from build123d import *

# Parameters (mm, degrees)
F0_R        = 50.8
F1_DEPTH    = 63.5
F2_T1_DEPTH = 128.3697077416
F2_T3_DEPTH = 128.3697077416
F2_T5_DEPTH = 78.8079500043


# Not quite as in the source:
# - a fillet or chamfer that OpenCascade refuses, or shapes differently, is made with other operations: its cross-section is extruded or revolved along the edge and cut away or added


with BuildPart() as f1:
    # F0 (on Top) → F1 (new body)
    with BuildSketch(Plane.XY):
        Polygon((-88.9, -51.326438931), (0, -102.6528778619), (88.9, -51.326438931), (88.9, 51.326438931), (0, 102.6528778619), (-88.9, 51.326438931), align=None)
        Circle(F0_R, mode=Mode.SUBTRACT)
    extrude(amount=F1_DEPTH)

    # F2: chamfer of 5 on 6 edges, made by hand

    # F2_s2 → F2_t1 (cut)
    with BuildSketch(Plane(origin=(55.5857139903, -32.0924269354, 0), x_dir=(0, 0, 1), z_dir=(-0.8660254038, 0.5, 0))):
        Polygon((58.5, 88.9), (63.5, 83.9), (63.5, 88.9), align=None)
        Polygon((5, 88.9), (0, 83.9), (0, 88.9), align=None)
    extrude(amount=F2_T1_DEPTH, mode=Mode.SUBTRACT)

    # F2_s4 → F2_t3 (cut)
    with BuildSketch(Plane(origin=(55.5857139903, 32.0924269354, 0), x_dir=(0, 0, 1), z_dir=(-0.8660254038, -0.5, 0))):
        Polygon((58.5, 88.9), (63.5, 83.9), (63.5, 88.9), align=None)
        Polygon((5, 88.9), (0, 83.9), (0, 88.9), align=None)
    extrude(amount=F2_T3_DEPTH, mode=Mode.SUBTRACT)

    # F2_s6 → F2_t5 (cut)
    with BuildSketch(Plane.XY.offset(-7.6539750021)):
        Polygon((-88.9, 48.439687585), (-86.4, 52.7698146039), (-88.9, 51.326438931), align=None)
        Polygon((88.9, 48.439687585), (86.4, 52.7698146039), (88.9, 51.326438931), align=None)
    extrude(amount=F2_T5_DEPTH, mode=Mode.SUBTRACT)


solid = f1.part
Work out the finished part from the listing and answer in its coordinate system (mm). Give positions to 0.01 mm unless a question says otherwise; leave off trailing zeros. Write each loop counter-clockwise with the first axis right and the second up, starting at its lowest first coordinate (ties: lowest second). Pieces come first, ordered by that corner, then holes.
Q1. The part is cut by section A-A on z = 48. Give the vertices of the cut face in (x, y).
Answer:
outline: (-88.9, -51.33) - (0, -102.65) - (88.9, -51.33) - (88.9, 48.44) - (86.4, 52.77) - (0, 102.65) - (-86.4, 52.77) - (-88.9, 48.44) - close; hole circle Ø101.6 at (0, 0)
Q2. Straight lines are drawn through the part: L1, parallel to Y at x = 0, z = 26; L2, parallel to Y at x = 39, z = 59; L3, parallel to X at y = 31, z = 54.5. For each, find the intervals that lie inside material, in ascending order.
Answer:
L1: y = -102.65 to -50.8, 50.8 to 102.65
L2: y = -80.14 to -32.55, 32.55 to 79.56
L3: x = -88.9 to -40.24, 40.24 to 88.9
Q3. The part is cut by section C-C on x = -12.5. Give the vertices of the cut face in (y, z).
Answer:
outline: (-95.44, 0) - (-49.24, 0) - (-49.24, 63.5) - (-95.44, 63.5) - close; (49.24, 0) - (89.66, 0) - (95.44, 5) - (95.44, 58.5) - (89.66, 63.5) - (49.24, 63.5) - close
Q4. For a pull along Y with two mould halves and no side action, classify faces 1 (the face through (43.805, 77.362, 31.376)), 2 (the face through (-11.012, -49.592, 31.306)), 3 (the face through (-88.9, -1, 31)) as released by +Y, released by -Y, zero draft, split by the parting line, or undercut.
Answer:
face 1: released by +Y
face 2: undercut
face 3: zero draft
Q5. The part is cut by section B-B on y = 0. Give the vertices of the cut face in (x, z), and give its area (3 significant figures).
Answer:
outline: (-88.9, 0) - (-50.8, 0) - (-50.8, 63.5) - (-88.9, 63.5) - close; (50.8, 0) - (88.9, 0) - (88.9, 63.5) - (50.8, 63.5) - close
area: 4,840 mm2
Q6. Given pin 1 (1.5 mm diameter, centred on x = -41, z = 39, fed in from -Y); pin 2 (12 mm diameter, centred on x = -0.5, z = 31.5, fed in from -Y); pin 3 (1 mm diameter, centred on y = 66, z = 35, fed in from +X), each flat-ended and moving along its own axis, determine where each tip first touches the part or whether it passes through.
Answer:
pin 1: stops at y = -79.41
pin 2: stops at y = -102.65
pin 3: stops at x = 64.35
Q7. The part is cut by section D-D on y = 60.5. Give the vertices of the cut face in (x, z), and give its area (3 significant figures).
Answer:
outline: (-73.01, 5) - (-63.01, 0) - (63.01, 0) - (73.01, 5) - (73.01, 58.5) - (63.01, 63.5) - (-63.01, 63.5) - (-73.01, 58.5) - close
area: 9,170 mm2
